Here's the drawing with two shaded views (mm, measured from the low corner). I have some questions. Coordinates: 2 decimals unless noted, no trailing zeros. Loops run counter-clockwise (first coordinate to the right, second up) from the corner with the lowest first, then second, coordinate; pieces in that order, holes last. Notation, with made-up numbers: (86, -35.5) -> (138, -35.5) arc R25 ccw to (138, -17.5) -> close; hole circle Ø8 at (74.5, 13). An arc over 180 degrees is marked (long way). Answer as a JSON object with one key per item and string values. Group by question number.
Q1. I want a section at B-B on y = 42.5. Write out the boundary of the cut face in (x, z), then the cut area to 3 significant figures.
Q2. I want a section at C-C on x = 12.5. Write out the boundary of the cut face in (y, z).
Q3. I need wall thicknesses on line 1 (Z direction, x = 7, y = 38.5); line 2 (X direction, y = 40, z = 35); line 3 (Z direction, x = 9.25, y = 44). Which ranges of each line are inside material? Lowest first, please.
Q4. I want a section at A-A on z = 7. Write out the boundary of the cut face in (x, y).
Q5. I want a section at D-D on z = 38.5. Write out the boundary of the cut face in (x, y), then the cut area to 3 significant figures.
Q6. I'm going to push a flat-ended pin straight in: pin 1 (4.5 mm diameter, centred on x = 7, z = 35, fed in from +Y). Where does the tip first touch, or does it pass through?
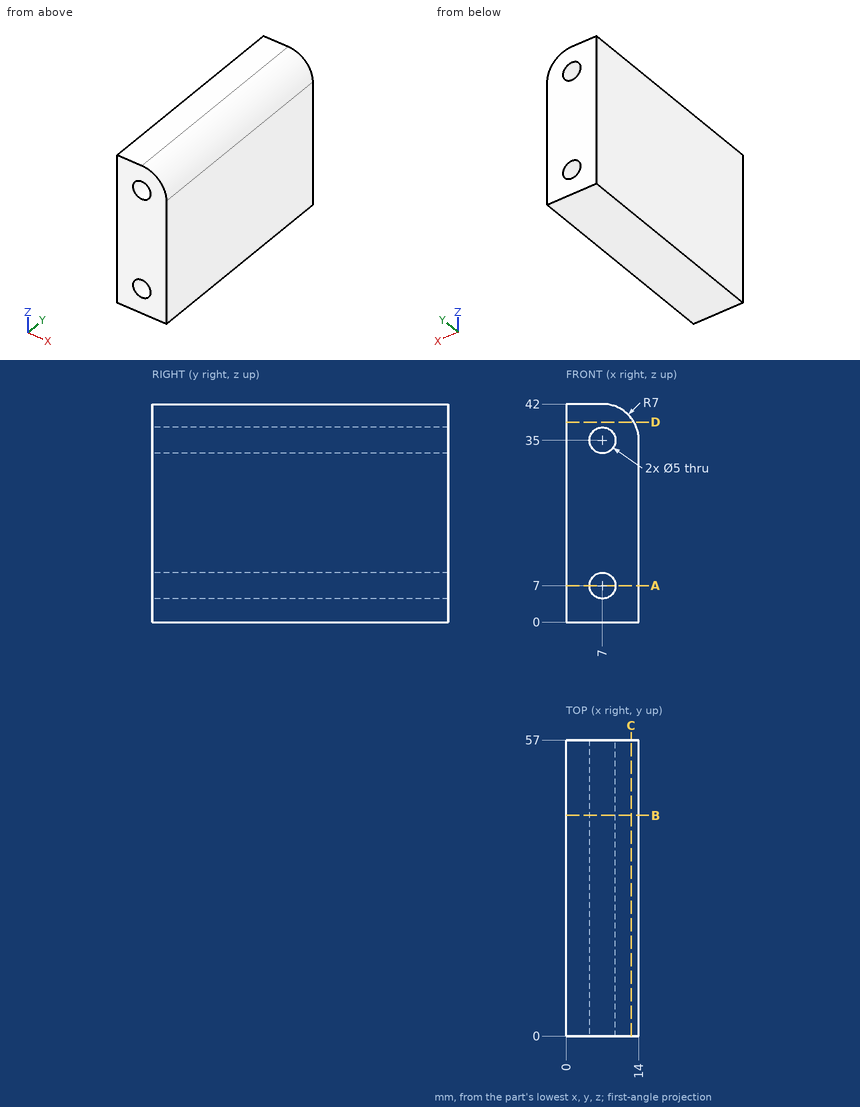
Result set:
{
 "1": {"outline": "(0, 0) -> (14, 0) -> (14, 35) arc R7 ccw to (7, 42) -> (0, 42) -> close; hole circle Ø5 at (7, 7); hole circle Ø5 at (7, 35)", "area": "538 mm²"},
 "2": {"outline": "(0, 0) -> (57, 0) -> (57, 39.33) -> (0, 39.33) -> close"},
 "3": {"line 1": "z = 0 to 4.5, 9.5 to 32.5, 37.5 to 42", "line 2": "x = 0 to 4.5, 9.5 to 14", "line 3": "z = 0 to 5.91, 8.09 to 33.91, 36.09 to 41.63"},
 "4": {"outline": "(0, 0) -> (4.5, 0) -> (4.5, 57) -> (0, 57) -> close; (9.5, 0) -> (14, 0) -> (14, 57) -> (9.5, 57) -> close"},
 "5": {"outline": "(0, 0) -> (13.06, 0) -> (13.06, 57) -> (0, 57) -> close", "area": "745 mm²"},
 "6": {"pin 1": "passes through"}
}
